The model under review builds one solid part; all positions refer to its coordinate system, in mm. Face numbers are marked on the shaded views. A direction names the side the tool comes from. Round coordinates to 2 decimals unless told otherwise and drop trailing zeros. Write each loop counter-clockwise with the first axis right and the second up, starting at its lowest first coordinate (ties: lowest second). Pieces come first, ordered by that corner, then holes. Notation, with made-up numbers: M 37.25,24 L 65.25,24 A17 cw 65.25,46 Z; hole C 72.25,56.5 d5. An arc over 180 degrees is marked long. Write item = value, one per line. Start each with the question number.
Item 1: Take a section at B-B, the plane z = 0. Give the boundary of the cut face in (x, y).
Item 2: To check wall thickness, follow line 1 along Z through (x, y) = (0, -2.75); line 2 along Z through (x, y) = (0, 0.5); line 3 along Y through (x, z) = (-1.75, -5.25). State the ranges of each line that lie inside material, in increasing order.
Item 3: Take a section at D-D, the plane z = 5.5. Give the boundary of the cut face in (x, y), plus the area to 3 significant figures.
Item 4: For pin 1 Ø8 at (x, z) = (0, 0) entering from +Y; pin 2 Ø1.5 at (x, y) = (-4, -3.5) entering from -Z; pin 3 Ø1 at (x, y) = (0.5, -8) entering from -Z; pin 4 Ø1.5 at (x, y) = (1, 1) entering from -Z, all flat-tipped, find the tip position at first contact; note any pin that passes through.
Item 5: Tool access review of the marked faces 5 and 6: name each direction out of +Z, -Z, +X, -X, +Y, -Y from which nothing blocks a thin tool from reaching the whole face with its end or side.
Item 6: Take a section at A-A, the plane x = 0. Give the boundary of the cut face in (y, z).
Item 7: The part is to be moulded in two halves that separate along Z. For the marked faces 1, 2, 3 and 4, say which applies: +Z half, -Z half, draft (parallel to the pull), parting line (faces both ways), or undercut.
Item 8: Take a section at C-C, the plane y = -0.5. Give the boundary of the cut face in (x, z).
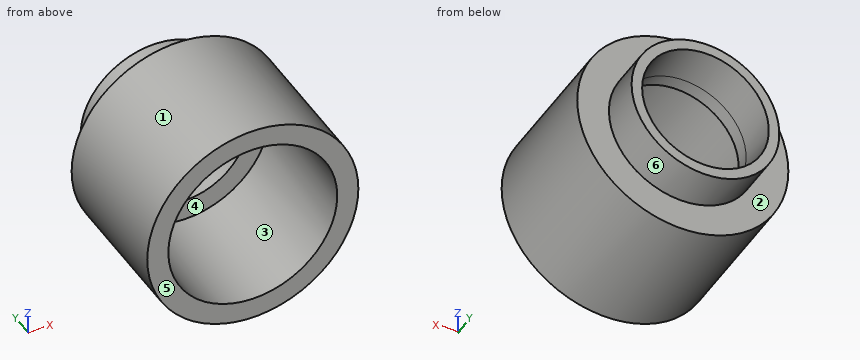
from build123d import *

# Parameters (mm, degrees)
F0_R          = 7.5
F0_R_2        = 6
F1_DEPTH      = 10
F0_R_3        = 5.25
F2_DEPTH      = 1
F0_R_4        = 4.5
F3_DEPTH      = 1
F3_DEPTH_BACK = 3


with BuildPart() as f1:
    # F0 (on Front) → F1 (new body)
    with BuildSketch(Plane.XZ):
        Circle(F0_R)
        Circle(F0_R_2, mode=Mode.SUBTRACT)
    extrude(amount=F1_DEPTH)

    # F0 (on Front) → F2 (join)
    with BuildSketch(Plane.XZ):
        Circle(F0_R_2)
        Circle(F0_R_3, mode=Mode.SUBTRACT)
    extrude(amount=F2_DEPTH)

    # F0 (on Front) → F3 (join, two sides)
    with BuildSketch(Plane.XZ) as f3_sk:
        Circle(F0_R_3)
        Circle(F0_R_4, mode=Mode.SUBTRACT)
    extrude(amount=F3_DEPTH)
    extrude(f3_sk.sketch, amount=-F3_DEPTH_BACK)


solid = f1.part
Response values:
q1.outline = M -7.5,-10 L -6,-10 L -6,-1 L -4.5,-1 L -4.5,3 L -5.25,3 L -5.25,0 L -7.5,0 Z; M 4.5,-1 L 6,-1 L 6,-10 L 7.5,-10 L 7.5,0 L 5.25,0 L 5.25,3 L 4.5,3 Z
q2.line_1 = -7.5 to -6, 6 to 7.5
q2.line_2 = -5.25 to -4.5, 4.5 to 5.25
q2.line_3 = -1 to 0
q3.outline = M -5.1,-10 L -2.4,-10 L -2.4,-1 L 2.4,-1 L 2.4,-10 L 5.1,-10 L 5.1,0 L -5.1,0 Z
q3.area = 58.8 mm2
q4.pin_1 = through
q4.pin_2 = -6.76
q4.pin_3 = -7.5
q4.pin_4 = -5.24
q5.face_5 = +Z, -Z, +X, -X, -Y
q5.face_6 = +Y
q6.outline = M -10,-7.5 L 0,-7.5 L 0,-5.25 L 3,-5.25 L 3,-4.5 L -1,-4.5 L -1,-6 L -10,-6 Z; M -10,6 L -1,6 L -1,4.5 L 3,4.5 L 3,5.25 L 0,5.25 L 0,7.5 L -10,7.5 Z
q7.face_1 = parting line
q7.face_2 = draft
q7.face_3 = undercut
q7.face_4 = undercut
q8.outline = C 0,0 d15; hole C 0,0 d9
